```python
from build123d import *

# Parameters (mm, degrees)
SKETCH_2_R            = 2.25
CUT_EXTRUDE_673_DEPTH = 45.270136661
SKETCH_2_3_R          = 3.55
CUT_EXTRUDE_707_DEPTH = 5


with BuildPart() as part:
    # Sketch 278 → Revolve 1 (revolve)
    with BuildSketch(Plane.XY, mode=Mode.PRIVATE) as revolve_1_sk:
        Polygon((17.15, 9), (30.65, 9), (30.65, 0), (18.65, 0), (18.65, 7), (17.15, 7), align=None)
    revolve(revolve_1_sk.sketch.rotate(Axis((0, 23.662648221, 0), (0, -1, 0)), 90), axis=Axis((0, 23.662648221, 0), (0, -1, 0)))

    # Sketch 2 → Cut-Extrude 673 (cut, through all)
    with BuildSketch(Plane(origin=(0, 9, 0), x_dir=(1, 0, 0), z_dir=(0, 1, 0))):
        with Locations(Location((0, 24.65, 0), (0, 0, 270))):
            Circle(SKETCH_2_R)
        with Locations(Location((21.347526203, -12.325, 0), (0, 0, 270))):
            Circle(SKETCH_2_R)
        with Locations(Location((-21.347526203, -12.325, 0), (0, 0, 270))):
            Circle(SKETCH_2_R)
    extrude(amount=-CUT_EXTRUDE_673_DEPTH, mode=Mode.SUBTRACT)

    # Sketch 2_3 → Cut-Extrude 707 (cut)
    with BuildSketch(Plane(origin=(0, 9, 0), x_dir=(1, 0, 0), z_dir=(0, 1, 0))):
        with Locations(Location((0, 24.65, 0), (0, 0, 270))):
            Circle(SKETCH_2_3_R)
        with Locations(Location((21.347526203, -12.325, 0), (0, 0, 270))):
            Circle(SKETCH_2_3_R)
        with Locations(Location((-21.347526203, -12.325, 0), (0, 0, 270))):
            Circle(SKETCH_2_3_R)
    extrude(amount=-CUT_EXTRUDE_707_DEPTH, mode=Mode.SUBTRACT)


solid = part.part
```
Here's how the part is built. I have some questions about the finished solid (model axes, mm). A direction names the side the tool comes from. Round coordinates to 2 decimals unless told otherwise and drop trailing zeros. Write each loop counter-clockwise with the first axis right and the second up, starting at its lowest first coordinate (ties: lowest second). Pieces come first, ordered by that corner, then holes. Notation, with made-up numbers: M -18,1 L 37,1 A27 ccw 37,40 Z; hole C -1.5,24.5 d1. An arc over 180 degrees is marked long. Answer as CSV lines item,"result". Start each with the question number.
1. I'm going to push flat-ended pins straight in: pin 1 Ø2 at (y, z) = (2, -6) entering from +X; pin 2 Ø5.5 at (x, z) = (-22, 12) entering from +Y; pin 3 Ø2 at (x, z) = (-0.5, -24.5) entering from +Y. Where does each tip first touch, or does it pass through?
2. Suppose I cut it at D-D on y = 8. Write out the boundary of the cut face in (x, z) (3 decimals), then the cut area to 3 significant figures.
3. Suppose I cut it at C-C on x = 8. Write out the boundary of the cut face in (y, z), then the cut area to 3 significant figures.
4. On a 3-axis mill with a long thin cutter (end or side, diameter ignored), from which of +Z, -Z, +X, -X, +Y, -Y can I reach the whole of each face in a straight line? I mean faces 1 (the flat face through (13, 9, -13)), 2 (the flat face through (21, 4, 15)), 3 (the flat face through (16.5, 7, 5.4)). Say none if no direction works.
5. Suppose I cut it at B-B on z = 0. Write out the boundary of the cut face in (x, y).
6. I need wall thicknesses on probe 1 along X at (y, z) = (8.3, 0); probe 2 along X at (y, z) = (5, 0); probe 3 along Z at (x, y) = (-2, 5.75). Which ranges of each line are inside material? Lowest first, please.
7. Suppose I cut it at A-A on x = 0. Write out the boundary of the cut face in (y, z).
Check result:
1,pin 1,"stops at x = 30.24"
1,pin 2,"stops at y = 4"
1,pin 3,"passes through"
2,outline,"C 0,0 d61.3; hole C -21.348,12.325 d7.1; hole C 0,0 d34.3; hole C 0,-24.65 d7.1; hole C 21.348,12.325 d7.1"
2,area,"1,910 mm2"
3,outline,"M 0,-29.59 L 9,-29.59 L 9,-15.17 L 7,-15.17 L 7,-16.85 L 0,-16.85 Z; M 0,16.85 L 7,16.85 L 7,15.17 L 9,15.17 L 9,29.59 L 0,29.59 Z"
3,area,"236 mm2"
4,face 1,"+Z, -Z, +X, -X, +Y"
4,face 2,"+Y"
4,face 3,"-Y"
5,outline,"M -30.65,0 L -18.65,0 L -18.65,7 L -17.15,7 L -17.15,9 L -30.65,9 Z; M 17.15,7 L 18.65,7 L 18.65,0 L 30.65,0 L 30.65,9 L 17.15,9 Z"
6,probe 1,"x = -30.65 to -17.15, 17.15 to 30.65"
6,probe 2,"x = -30.65 to -18.65, 18.65 to 30.65"
6,probe 3,"z = -30.58 to -27.58, -21.72 to -18.54, 18.54 to 30.58"
7,outline,"M 0,-30.65 L 9,-30.65 L 9,-28.2 L 4,-28.2 L 4,-26.9 L 0,-26.9 Z; M 0,-22.4 L 4,-22.4 L 4,-21.1 L 9,-21.1 L 9,-17.15 L 7,-17.15 L 7,-18.65 L 0,-18.65 Z; M 0,18.65 L 7,18.65 L 7,17.15 L 9,17.15 L 9,30.65 L 0,30.65 Z"
